Here's how the part is built. I have some questions about the finished solid (model axes, mm). A direction names the side the tool comes from. Give positions to 0.01 mm unless a question says otherwise; leave off trailing zeros. Order: outer loops, then holes, each group sorted by start corner. A loop starts at its lowest first (then second) coordinate and runs counter-clockwise, first axis right, second up.
from build123d import *

# Parameters (mm, degrees)
F1_DEPTH = 25.4


with BuildPart() as f1:
    # F0 (on Front) → F1 (new body, symmetric)
    with BuildSketch(Plane.XZ):
        Polygon((-1.625, -0.5625), (1.625, -0.5625), (1.625, 0.5625), (0.875, 0.5625), (-1.625, 0.5625), align=None)
        with BuildLine():
            Line((0.875, 0.5625), (1.625, 0.5625))
            Line((1.625, 0.5625), (1.625, 0.8755))
            ThreePointArc((1.625, 0.8755), (1.739421, 1.235964), (2.04079, 1.464445))
            Line((2.04079, 1.464445), (2.04079, 2.234491))
            ThreePointArc((2.04079, 2.234491), (1.206379, 1.770755), (0.875, 0.8755))
            Line((0.875, 0.8755), (0.875, 0.5625))
        make_face()
        with BuildLine():
            ThreePointArc((2.25, 2.2505), (2.145089, 2.246492), (2.04079, 2.234491))
            Line((2.04079, 2.234491), (2.04079, 1.464445))
            ThreePointArc((2.04079, 1.464445), (2.143853, 1.49142), (2.25, 1.5005))
            Line((2.25, 1.5005), (3.375, 1.5005))
            Line((3.375, 1.5005), (3.375, 2.2505))
            Line((3.375, 2.2505), (2.25, 2.2505))
        make_face()
        with BuildLine():
            Line((2.04079, 2.4375), (2.04079, 2.234491))
            ThreePointArc((2.04079, 2.234491), (2.145089, 2.246492), (2.25, 2.2505))
            Line((2.25, 2.2505), (3.375, 2.2505))
            Line((3.375, 2.2505), (3.375, 1.5005))
            Line((3.375, 1.5005), (2.25, 1.5005))
            ThreePointArc((2.25, 1.5005), (2.143853, 1.49142), (2.04079, 1.464445))
            Line((2.04079, 1.464445), (2.04079, 1.3125))
            Line((2.04079, 1.3125), (5.04079, 1.3125))
            Line((5.04079, 1.3125), (5.04079, 2.4375))
            Line((5.04079, 2.4375), (2.04079, 2.4375))
        make_face()
    extrude(amount=F1_DEPTH, both=True)


solid = f1.part
Q1. I need wall thicknesses on L1, parallel to X at y = 13, z = 0.9; L2, parallel to Z at x = 3.75, y = 16; L3, parallel to Z at x = 0.5, y = 10.5. Which ranges of each line are inside material? Lowest first, please.
Filled sheet:
L1: x = 0.88 to 1.63
L2: z = 1.31 to 2.44
L3: z = -0.56 to 0.56
Q2. If we section it at C-C on x = 3.5: List the corners of the cut face in (y, z) for me, plus the area to 4 significant figures.
Filled sheet:
outline: (-25.4, 1.31) - (25.4, 1.31) - (25.4, 2.44) - (-25.4, 2.44) - close
area: 57.15 mm2
Q3. If we section it at B-B on z = -0.05: List the corners of the cut face in (x, y) for me (3 decimals).
Filled sheet:
outline: (-1.625, -25.4) - (1.625, -25.4) - (1.625, 25.4) - (-1.625, 25.4) - close
Q4. I'm going to push flat-ended pins straight in: P1, Ø1.2, axis at x = 0, y = -8, coming from the +Z side; P2, Ø3.5, axis at x = 4, y = 4, coming from the -Z side. Where does each tip first touch, or does it pass through?
Filled sheet:
P1: stops at z = 0.56
P2: stops at z = 1.31
Q5. For faces 1 (the face through (4, 0, 2.438)), 2 (the face through (1.625, 0, 0)), 3 (the face through (0, 0, 0.562)), which set-ups out of +Z, -Z, +X, -X, +Y, -Y let a thin tool reach every point of the face, with its end or its side?
Filled sheet:
face 1: +Z, +X, -X, +Y, -Y
face 2: -Z, +X, +Y, -Y
face 3: +Z, -X, +Y, -Y
Q6. Thinking about a two-plate mould opening in Z: for faces 4 (the face through (4, 0, 1.312)), 5 (the face through (1.215, -0.356, 1.781)), 6 (the face through (1.4, 25.4, 1.1)), which applies, released by +Z, released by -Z, zero draft, split by the parting line, or undercut?
Filled sheet:
face 4: released by -Z
face 5: released by +Z
face 6: zero draft
